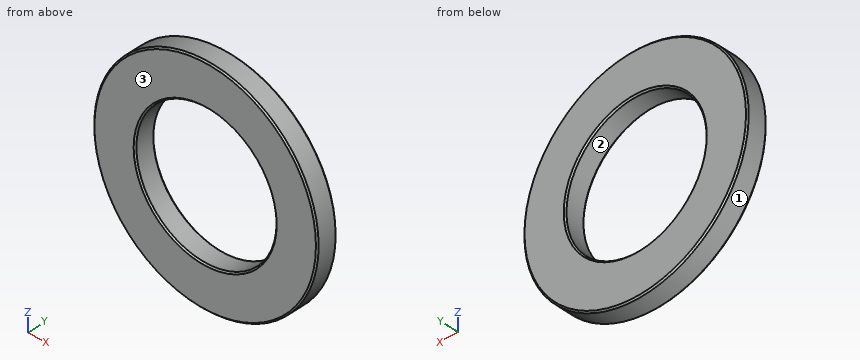
from build123d import *

# Parameters (mm, degrees)
PROFILES_R    = 8
PROFILES_R_2  = 5
PROFILE_DEPTH = 1.5
OUTERC_SIZE   = 0.1
INNERC_SIZE   = 0.1


with BuildPart() as part:
    # ProfileS → Profile (new body)
    with BuildSketch(Plane(origin=(0, 0, 0), x_dir=(1, 0, 0), z_dir=(0, 1, 0))):
        Circle(PROFILES_R)
        Circle(PROFILES_R_2, mode=Mode.SUBTRACT)
    extrude(amount=PROFILE_DEPTH)

    # OuterC
    outerc_edges = [part.edges().sort_by_distance(p)[0] for p in [
        (-8, 0, 0),
        (-8, 1.5, 0),
    ]]
    chamfer(outerc_edges, length=OUTERC_SIZE)

    # InnerC
    innerc_edges = [part.edges().sort_by_distance(p)[0] for p in [
        (-5, 0, 0),
        (-5, 1.5, 0),
    ]]
    chamfer(innerc_edges, length=INNERC_SIZE)


solid = part.part
Can you work these out from the model? Positions are in its coordinate system, mm. Face numbers are marked on the shaded views. Coordinates: 2 decimals unless noted, no trailing zeros. Write each loop counter-clockwise with the first axis right and the second up, starting at its lowest first coordinate (ties: lowest second). Pieces come first, ordered by that corner, then holes. Notation, with made-up numbers: (68.5, -15) -> (94.5, -15) arc R27 cw to (94.5, 16) -> close; hole circle Ø11 at (-24.75, 10). An arc over 180 degrees is marked (long way). Answer as CSV lines item,"result".
1) If we mould it in two halves opening along Z, with no side actions, what happens to the marked faces 1, 2 and 3? For each: +Z half, -Z half, draft (parallel to the pull), parting line (faces both ways), or undercut.
Check result:
face 1,"parting line"
face 2,"undercut"
face 3,"draft"
2) If I drill on line 1 (Z direction, x = 0, y = 1); line 2 (X direction, y = 1.45, z = 2.5), over which ranges is the centre line in solid material (lowest first)? Write a range as from..to.
Check result:
line 1,"-8..-5, 5..8"
line 2,"-7.55..-4.39, 4.39..7.55"
3) If we section it at A-A on x = 0: Please give me the cut outline in (y, z).
Check result:
outline,"(0, -7.9) -> (0.1, -8) -> (1.4, -8) -> (1.5, -7.9) -> (1.5, -5.1) -> (1.4, -5) -> (0.1, -5) -> (0, -5.1) -> close; (0, 5.1) -> (0.1, 5) -> (1.4, 5) -> (1.5, 5.1) -> (1.5, 7.9) -> (1.4, 8) -> (0.1, 8) -> (0, 7.9) -> close"
4) If we section it at C-C on y = 0.3: Please give me the cut outline in (x, z).
Check result:
outline,"circle Ø16 at (0, 0); hole circle Ø10 at (0, 0)"
5) If we section it at B-B on z = 0: Please give me the cut outline in (x, y), then the cut area to 3 significant figures.
Check result:
outline,"(-8, 0.1) -> (-7.9, 0) -> (-5.1, 0) -> (-5, 0.1) -> (-5, 1.4) -> (-5.1, 1.5) -> (-7.9, 1.5) -> (-8, 1.4) -> close; (5, 0.1) -> (5.1, 0) -> (7.9, 0) -> (8, 0.1) -> (8, 1.4) -> (7.9, 1.5) -> (5.1, 1.5) -> (5, 1.4) -> close"
area,"8.96 mm²"
